Part model, mm, in its own coordinate system. Face numbers are marked on the shaded views. Give positions to 0.01 mm unless a question says otherwise; leave off trailing zeros. Loops run counter-clockwise (first coordinate to the right, second up) from the corner with the lowest first, then second, coordinate; pieces in that order, holes last. Notation, with made-up numbers: (60, 59) -> (70, 59) arc R14 ccw to (70, 68) -> close; hole circle Ø11 at (-36.5, -12.5). An arc over 180 degrees is marked (long way). Write item = value, one per line.
Autodesk Inventor part; units mm, degrees
ref_plane "Plano de trabajo1" through (35, 60.0697, 0) normal (1, 0, 0) x (0, 1, 0)
ref_plane "Plano de trabajo10" through (35, 15, 0) normal (1, 0, 0) x (0, 1, 0)
ref_plane "XZ Plane" through (0, 0, 0) normal (0, 1, 0) x (-1, 0, 0)
sketch "Boceto1" plane through (0, 0, 0) normal (0, 0, 1) x (1, 0, 0)
  line L0 (0, 0) -> (-32.5, 0)
  line L1 (0, 0) -> (0, 70)
  line L2 (0, 70) -> (-35, 70)
  line L3 (-35, 70) -> (-35, 5)
  arc A0 (-35, 5) -> (-32.5, 0) centre (-28.75, 5) ccw
  dimension "d0" = 32.5
  dimension "d1" = 70
  dimension "d2" = 35
  dimension "d3" = 65
revolve "Revolución1" add sketch "Boceto1" angle 360 about axis through (0, 0, 0) along (0, 1, 0)
shell "Vaciado1" thickness 3 removed faces 1 at (-0.2748, 70, -9.3581)
sketch "Boceto2" plane through (0, 0, 0) normal (0, 0, 1) x (1, 0, 0)
  line L0 (35, 5) -> (35, 70)
  line L1 (32, 5) -> (32, 70)
  line L2 (35, 60.0697) -> (60, 60.0697)
  arc A0 (66.5079, 49.9877) -> (60, 60.0697) centre (54.5227, 49.3927) ccw
  line L3 (66.5079, 49.9877) -> (35, 15)
  point P0 (0, 0)
  dimension "d10" = 25
  dimension "d11" = 12
  dimension "d12" = 12
ref_plane "Plano de trabajo1" through (35, 60.0697, 0) normal (1, 0, 0) x (0, 1, 0)
sketch "Boceto3" plane through (35, 60.0697, 0) normal (1, 0, 0) x (0, 1, 0)
  ellipse E0 centre (0, 0) end of major axis (-4, 0) minor radius 6
  point P0 (-60.0697, 0)
  dimension "d14" = 4
  dimension "d15" = 6
ref_plane "Plano de trabajo10" through (35, 15, 0) normal (1, 0, 0) x (0, 1, 0)
sketch "Boceto8" plane through (35, 15, 0) normal (1, 0, 0) x (0, 1, 0)
  ellipse E0 centre (0, 0) end of major axis (-3, 0) minor radius 5
  point P0 (-15, 0)
  dimension "d23" = 5
  dimension "d24" = 3
fillet "Empalme1" radius 2 1 edges at (35, 70, 0)
sketch "Boceto9" plane through (0, 0, 0) normal (0, -1, 0) x (1, 0, 0)
  circle A0 centre (0, 0) radius 32.5
  circle A1 centre (0, 0) radius 31
  dimension "d26" = 65
  dimension "d27" = 62
properties part number "Taza Juan Molina"
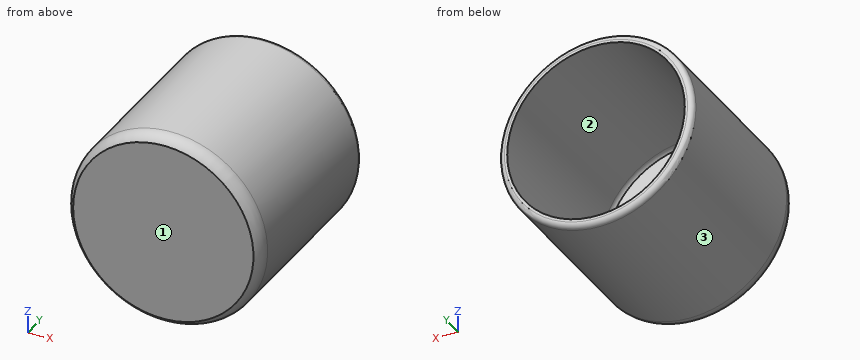
1) Slice it at B-B, the plane x = 0. List the corners of the cut face in (y, z).
Resolved:
outline = (0, -32.5) arc R6.25 ccw to (5, -35) -> (68, -35) arc R2 ccw to (70, -33) -> (70, -32) -> (5, -32) arc R3.25 cw to (3, -31.31) -> (3, 31.31) arc R3.25 cw to (5, 32) -> (70, 32) -> (70, 33) arc R2 ccw to (68, 35) -> (5, 35) arc R6.25 ccw to (0, 32.5) -> close
2) Pull direction X, two halves, no side cores. Call the marked faces 1, 2 and 3: pulls with the +X half, pulls with the -X half, needs draft (parallel to the pull), parting line crosses it, or undercut.
Resolved:
face_1 = needs draft
face_2 = undercut
face_3 = parting line crosses it
3) Drill centre lines: line 1 along Z through (x, y) = (0, 46); line 2 along Y through (x, z) = (-11, -1). Where is each one in solid material? Low to high. Write a range as [from, to].
Resolved:
line_1 = [-35, -32], [32, 35]
line_2 = [0, 3]
4) Drop flat-ended pins along their axis: P1, Ø2, axis at x = 20.5, y = 11.5, coming from the -Z side; P2, Ø10, axis at x = 3.5, y = 56, coming from the +Z side; P3, Ø6, axis at y = 54.5, z = -8.5, coming from the -X side. Give the stop position or say it passes through.
Resolved:
P1 = -29.06
P2 = 35
P3 = -34.57
5) Slice it at A-A, the plane z = 0. List the corners of the cut face in (x, y).
Resolved:
outline = (-35, 5) arc R6.25 ccw to (-32.5, 0) -> (32.5, 0) arc R6.25 ccw to (35, 5) -> (35, 68) arc R2 ccw to (33, 70) -> (32, 70) -> (32, 5) arc R3.25 cw to (31.31, 3) -> (-31.31, 3) arc R3.25 cw to (-32, 5) -> (-32, 70) -> (-33, 70) arc R2 ccw to (-35, 68) -> close
6) Slice it at C-C, the plane y = 41.5. List the corners of the cut face in (x, z).
Resolved:
outline = circle Ø70 at (0, 0); hole circle Ø64 at (0, 0)
